Here's how the part is built. I have some questions about the finished solid (model axes, mm). A direction names the side the tool comes from. Round coordinates to 2 decimals unless told otherwise and drop trailing zeros. Order: outer loops, then holes, each group sorted by start corner. A loop starts at its lowest first (then second) coordinate and runs counter-clockwise, first axis right, second up. Notation, with made-up numbers: (82, -25.75) -> (140, -25.75) arc R16 cw to (140, -1.75) -> close; hole circle Ø8 at (-5.75, -29.75). An arc over 180 degrees is marked (long way). Use a Markdown table: item, result. Add a question column.
(1) I want a section at C-C, the plane y = 5.4. Please give me the cut outline in (x, z), then the cut area to 3 significant figures.
(2) I want a section at B-B, the plane x = -24.5. Please give me the cut outline in (y, z), then the cut area to 3 significant figures.
(3) I want a section at A-A, the plane z = 5.25. Please give me the cut outline in (x, y).
(4) I'm going to push a flat-ended pin straight in: P1, Ø2, axis at x = -26, y = 5, coming from the +Z side. Where does the tip first touch, or does it pass through?
(5) If I drill on probe 1 along Y at (x, z) = (-24.5, 1.75); probe 2 along X at (y, z) = (3.3, 3); probe 3 along Z at (x, y) = (-27, 3.35), over which ranges is the centre line in solid material (lowest first)?
(6) Thinking about a two-plate mould opening in X: for faces 3 (the face through (-28.435, 5, 3)), 4 (the face through (-24, 5, -1)), 5 (the face through (-24, 6.888, 3)), which applies, pulls with the +X half, pulls with the -X half, needs draft (parallel to the pull), parting line crosses it, or undercut?
(7) On a 3-axis mill with a long thin cutter (end or side, diameter ignored), from which of +Z, -Z, +X, -X, +Y, -Y can I reach the whole of each face in a straight line? I mean faces 1 (the face through (-24, 5, 0)), 2 (the face through (-24.5, 7.6, 6)). Say none if no direction works.
from build123d import *

# Parameters (mm, degrees)
CROQUIS1_W              = 8
CROQUIS1_H              = 6
CROQUIS1_W_2            = 6
CROQUIS1_H_2            = 4
SALIENTE_EXTRUIR1_DEPTH = 6
CROQUIS3_W              = 8
CROQUIS3_H              = 6
SALIENTE_EXTRUIR2_DEPTH = 1


with BuildPart() as part:
    # Croquis1 → Saliente-Extruir1 (new body)
    with BuildSketch(Plane.XY):
        with Locations((-24.435275528, 4.888284157)):
            Rectangle(CROQUIS1_W, CROQUIS1_H)
        with Locations((-24.435275528, 4.888284157)):
            Rectangle(CROQUIS1_W_2, CROQUIS1_H_2, mode=Mode.SUBTRACT)
    extrude(amount=SALIENTE_EXTRUIR1_DEPTH)

    # Croquis3 → Saliente-Extruir2 (add)
    with BuildSketch(Plane(origin=(0, 0, 0), x_dir=(-1, 0, 0), z_dir=(0, 0, -1))):
        with Locations((24.435275528, 4.888284157)):
            Rectangle(CROQUIS3_W, CROQUIS3_H)
    extrude(amount=SALIENTE_EXTRUIR2_DEPTH)


solid = part.part
Taken from the geometry:
| question | item | result |
|---|---|---|
| 1 | outline | (-28.44, -1) -> (-20.44, -1) -> (-20.44, 6) -> (-21.44, 6) -> (-21.44, 0) -> (-27.44, 0) -> (-27.44, 6) -> (-28.44, 6) -> close |
| 1 | area | 20.0 mm2 |
| 2 | outline | (1.89, -1) -> (7.89, -1) -> (7.89, 6) -> (6.89, 6) -> (6.89, 0) -> (2.89, 0) -> (2.89, 6) -> (1.89, 6) -> close |
| 2 | area | 18.0 mm2 |
| 3 | outline | (-28.44, 1.89) -> (-20.44, 1.89) -> (-20.44, 7.89) -> (-28.44, 7.89) -> close; hole (-27.44, 2.89) -> (-21.44, 2.89) -> (-21.44, 6.89) -> (-27.44, 6.89) -> close |
| 4 | P1 | stops at z = 0 |
| 5 | probe 1 | y = 1.89 to 2.89, 6.89 to 7.89 |
| 5 | probe 2 | x = -28.44 to -27.44, -21.44 to -20.44 |
| 5 | probe 3 | z = -1 to 0 |
| 6 | face 3 | pulls with the -X half |
| 6 | face 4 | needs draft |
| 6 | face 5 | undercut |
| 7 | face 1 | +Z |
| 7 | face 2 | +Z, +X, -X, +Y, -Y |
